```python
from build123d import *

# Parameters (mm, degrees)
F0_W     = 52.6
F0_H     = 26.6
F0_W_2   = 51.8
F0_H_2   = 25.8
F1_DEPTH = 0.4
F2_DEPTH = 8
F3_R     = 4
F4_R     = 4.4
F5_R     = 1
F6_R     = 1.5


with BuildPart() as f1:
    # F0 (on Top) → F1 (new body)
    with BuildSketch(Plane.XY):
        Rectangle(F0_W, F0_H)
        Rectangle(F0_W_2, F0_H_2, mode=Mode.SUBTRACT)
        Rectangle(F0_W_2, F0_H_2)
    extrude(amount=F1_DEPTH)

    # F0 (on Top) → F2 (join)
    with BuildSketch(Plane.XY):
        Rectangle(F0_W, F0_H)
        Rectangle(F0_W_2, F0_H_2, mode=Mode.SUBTRACT)
    extrude(amount=F2_DEPTH)

    # F3
    f3_edges = [f1.edges().sort_by_distance(p)[0] for p in [
        (-25.9, 12.9, 4.2),
        (25.9, 12.9, 4.2),
        (25.9, -12.9, 4.2),
        (-25.9, -12.9, 4.2),
    ]]
    fillet(f3_edges, radius=F3_R)

    # F4
    f4_edges = [f1.edges().sort_by_distance(p)[0] for p in [
        (26.3, 13.3, 4),
        (26.3, -13.3, 4),
        (-26.3, 13.3, 4),
        (-26.3, -13.3, 4),
    ]]
    fillet(f4_edges, radius=F4_R)

    # F5
    f5_edges = [f1.edges().sort_by_distance(p)[0] for p in [
        (0, 12.9, 0.4),
    ]]
    fillet(f5_edges, radius=F5_R)

    # F6
    f6_edges = [f1.edges().sort_by_distance(p)[0] for p in [
        (0, -13.3, 0),
    ]]
    fillet(f6_edges, radius=F6_R)


solid = f1.part
```
Input: part model. Units: mm. Frame: model coordinates. A direction names the side the tool comes from. Coordinates: 2 decimals unless noted, no trailing zeros. Loops run counter-clockwise (first coordinate to the right, second up) from the corner with the lowest first, then second, coordinate; pieces in that order, holes last.
Q1. Mould query, pull axis Y, two halves, no side actions, for faces 3 (the flat face through (0, 0, 0)), 4 (the cylindrical face through (-0.31, 12.87, 0.45)), 5 (the flat face through (-25.9, 0, 5)). Classes: +Y half, -Y half, draft (parallel to the pull), parting line (faces both ways), or undercut.
Results are:
face 3: draft
face 4: +Y half
face 5: undercut
Q2. Line query: line 1 along X through (y, z) = (3.5, 3.25); line 2 along Y through (x, z) = (3, 3); line 3 along Z through (x, y) = (17, 3.75). Output: solid intervals per line, ascending.
Results are:
line 1: x = -26.3 to -25.9, 25.9 to 26.3
line 2: y = -13.3 to -12.9, 12.9 to 13.3
line 3: z = 0 to 0.4
Q3. Section C-C, the plane x = -11. Return the cut outline in (y, z), and give its area (3 significant figures).
Results are:
outline: (-13.3, 1.5) arc R1.5 ccw to (-11.8, 0) - (11.8, 0) arc R1.5 ccw to (13.3, 1.5) - (13.3, 8) - (12.9, 8) - (12.9, 1.4) arc R1 cw to (11.9, 0.4) - (-11.9, 0.4) arc R1 cw to (-12.9, 1.4) - (-12.9, 8) - (-13.3, 8) - close
area: 16.2 mm2
Q4. Contact query for a flat-ended pin moving along its axis: pin 1 (4 mm diameter, centred on x = -3.5, y = 7.5, fed in from +Z). Output: stop coordinate, or through.
Results are:
pin 1: stops at z = 0.4
Q5. Set-up query: faces 1 (the cylindrical face through (-25.045, 11.977, 4.704)), 2 (the flat face through (25.9, 0, 5)). Return all of +Z, -Z, +X, -X, +Y, -Y with unobstructed straight access to the full face (end or side cutting, diameter ignored); none if empty.
Results are:
face 1: +Z, -Z, -X, +Y
face 2: +Z
Q6. Section B-B, the plane y = -8. Return the cut outline in (x, z), and give its area (3 significant figures).
Results are:
outline: (-26.3, 1.5) arc R1.5 ccw to (-24.8, 0) - (24.8, 0) arc R1.5 ccw to (26.3, 1.5) - (26.3, 8) - (25.9, 8) - (25.9, 1.4) arc R1 cw to (24.9, 0.4) - (-24.9, 0.4) arc R1 cw to (-25.9, 1.4) - (-25.9, 8) - (-26.3, 8) - close
area: 26.6 mm2
Q7. Section A-A, the plane z = 3.5. Return the cut outline in (x, y), and give its area (3 significant figures).
Results are:
outline: (-26.3, -8.9) arc R4.4 ccw to (-21.9, -13.3) - (21.9, -13.3) arc R4.4 ccw to (26.3, -8.9) - (26.3, 8.9) arc R4.4 ccw to (21.9, 13.3) - (-21.9, 13.3) arc R4.4 ccw to (-26.3, 8.9) - close; hole (-25.9, -8.9) arc R4 ccw to (-21.9, -12.9) - (21.9, -12.9) arc R4 ccw to (25.9, -8.9) - (25.9, 8.9) arc R4 ccw to (21.9, 12.9) - (-21.9, 12.9) arc R4 ccw to (-25.9, 8.9) - close
area: 59.8 mm2
